Autodesk Inventor part; units mm, degrees
ref_plane "YZ Plane" through (0, 0, 0) normal (1, 0, 0) x (0, 1, 0)
ref_plane "XZ Plane" through (0, 0, 0) normal (0, 1, 0) x (-1, 0, 0)
ref_plane "XY Plane" through (0, 0, 0) normal (0, 0, 1) x (1, 0, 0)
sketch "Sketch1" plane through (0, 0, 0) normal (0, 0, 1) x (1, 0, 0)
  line L0 (0, 0) -> (25, 0)
  line L1 (25, 0) -> (25, 3)
  line L2 (25, 3) -> (0, 3)
  line L3 (0, 3) -> (0, 0)
  dimension "d0" = 25
  dimension "d1" = 3
extrude "Extrusion1" add sketch "Sketch1" along normal blind 450
sketch "Sketch2" plane through (0, 3, 0) normal (0, 1, 0) x (1, 0, 0)
  line L0 (0, 0) -> (0, -450)
  line L1 (0, 0) -> (250, 0)
  line L2 (250, 0) -> (250, -25)
  line L3 (250, -25) -> (0, -25)
  line L4 (0, -25) -> (0, 0)
  dimension "d4" = 250
  dimension "d5" = 25
extrude "Extrusion2" add sketch "Sketch2" along normal blind 3
sketch "Sketch3" plane through (0, 3, 450) normal (0, 1, 0) x (1, 0, 0)
  line L0 (0, 450) -> (0, 0)
  line L1 (0, 0) -> (250, 0)
  line L2 (250, 0) -> (250, 25)
  line L3 (250, 25) -> (0, 25)
  line L4 (0, 25) -> (0, 0)
  dimension "d8" = 250
  dimension "d9" = 25
extrude "Extrusion3" add sketch "Sketch3" along normal blind 3
sketch "Sketch4" plane through (0, 3, 0) normal (0, -1, 0) x (1, 0, 0)
  line L0 (250, 0) -> (0, 0)
  line L1 (250, 0) -> (225, 0)
  line L2 (225, 0) -> (225, 450)
  line L3 (225, 450) -> (250, 450)
  line L4 (250, 450) -> (250, 0)
  dimension "d12" = 25
  dimension "d13" = 450
extrude "Extrusion4" add sketch "Sketch4" along normal blind 3
sketch "Sketch5" plane through (0, 3, 25) normal (0, 1, 0) x (1, 0, 0)
  line L0 (0, 25) -> (0, -175)
  line L1 (0, 0) -> (0, -400)
  line L2 (0, -175) -> (250, -175)
  line L3 (250, -175) -> (250, -225)
  line L4 (250, -225) -> (0, -225)
  line L5 (0, -225) -> (0, -175)
  dimension "d16" = 200
  dimension "d17" = 250
  dimension "d18" = 50
extrude "Extrusion5" add sketch "Sketch5" along normal blind 3
sketch "Sketch6" plane through (0, 6, 0) normal (0, 1, 0) x (1, 0, 0)
  line L0 (25, -25) -> (0, -25)
  line L1 (0, 0) -> (0, -25)
  line L2 (25, -25) -> (0, -25)
  line L3 (0, -25) -> (0, 0)
  line L4 (0, 0) -> (25, 0)
  line L5 (25, 0) -> (25, -25)
  line L6 (25, -25) -> (0, 0)
  line L7 (225, 0) -> (25, 0)
  line L8 (25, 0) -> (0, -25)
  circle A0 centre (12.5, -12.5) radius 2.5
  line L9 (0, -450) -> (250, -450)
  line L10 (250, -425) -> (0, -425)
  line L11 (0, -450) -> (25, -450)
  line L12 (25, -450) -> (25, -425)
  line L13 (25, -425) -> (0, -425)
  line L14 (0, -425) -> (0, -450)
  line L15 (250, -450) -> (225, -450)
  line L16 (225, -450) -> (225, -425)
  line L17 (225, -425) -> (250, -425)
  line L18 (250, -425) -> (250, -450)
  line L19 (0, -450) -> (25, -425)
  line L20 (25, -450) -> (0, -425)
  line L21 (250, -450) -> (225, -425)
  line L22 (225, -425) -> (225, -250)
  line L23 (225, -450) -> (250, -425)
  circle A1 centre (237.5, -437.5) radius 2.5
  circle A2 centre (12.5, -437.5) radius 2.5
  line L24 (250, -25) -> (250, 0)
  line L25 (225, -25) -> (250, -25)
  line L26 (250, 0) -> (225, 0)
  line L27 (225, 0) -> (225, -25)
  line L28 (225, -25) -> (250, -25)
  line L29 (250, -25) -> (250, 0)
  line L30 (250, -25) -> (225, 0)
  line L31 (225, 0) -> (225, -25)
  line L32 (225, 0) -> (225, -25)
  line L33 (225, -25) -> (250, 0)
  circle A3 centre (237.5, -12.5) radius 2.5
  dimension "d21" = 5
  dimension "d22" = 5
  dimension "d23" = 5
  dimension "d24" = 5
extrude "Extrusion6" cut sketch "Sketch6" against normal blind 100 contours A0 L8 L6 | L6 L8 A0 | A0 L6 L8 | L8 L6 A0 | A3 L33 L30 | L30 L33 A3 | A3 L30 L33 | L33 L30 A3 | A2 L20 L19 | L19 L20 A2 | L20 L19 A2 | A2 L19 L20 | A1 L21 L23 | L23 L21 A1 | L21 L23 A1 | A1 L23 L21
sketch "Sketch7" plane through (0, 6, 25) normal (0, 1, 0) x (1, 0, 0)
  circle A0 centre (12.5, -200) radius 2.5
  line L0 (0, -175) -> (0, -225)
  line L1 (0, -225) -> (250, -225)
  circle A1 centre (237.5, -200) radius 2.5
  line L2 (250, -225) -> (250, -175)
  line L3 (250, -175) -> (0, -175)
  point P0 (0, 25)
  dimension "d27" = 5
  dimension "d28" = 12.5
  dimension "d29" = 25
  dimension "d30" = 5
  dimension "d31" = 12.5
  dimension "d32" = 25
extrude "Extrusion7" cut sketch "Sketch7" against normal blind 100 contours A0 | A1
thread "Thread1"
thread "Thread2"
thread "Thread3"
thread "Thread4"
thread "Thread5"
thread "Thread6"
sketch "Sketch8" plane through (0, 6, 25) normal (0, 1, 0) x (1, 0, 0)
  circle A0 centre (12.5, -200) radius 2.5
  circle A1 centre (237.5, -200) radius 2.5
  circle A2 centre (125, -200) radius 6.35
  line L0 (250, -225) -> (250, -175)
  point P0 (0, 25)
  dimension "d47" = 12.7
  dimension "d48" = 125
extrude "Extrusion8" cut sketch "Sketch8" against normal blind 10 contours A2
sketch "Sketch9" plane through (0, 6, 450) normal (0, 1, 0) x (1, 0, 0)
  circle A0 centre (125, 11.2801) radius 6.35
  line L0 (250, 0) -> (250, 25)
  point P0 (0, 450)
  dimension "d51" = 12.7
  dimension "d52" = 125
extrude "Extrusion9" cut sketch "Sketch9" against normal through all
thread "Thread7"
sketch "Sketch10" plane through (0, 3, 425) normal (0, 1, 0) x (1, 0, 0)
  line L0 (25, 425) -> (25, -25)
  line L1 (0, 425) -> (0, -25)
  line L2 (25, 0.3749) -> (0, 0.3749)
  line L3 (0, 0.3749) -> (0, 100.3749)
  line L4 (0, 100.3749) -> (25, 100.3749)
  line L5 (25, 100.3749) -> (25, 0.3749)
  circle A0 centre (12.5, 20.3749) radius 2.5
  circle A1 centre (12.5, 80.3749) radius 2.5
  point P0 (12.5, 0.3749)
  point P1 (12.5, 100.3749)
  dimension "d57" = 100
  dimension "d58" = 5
  dimension "d59" = 5
  dimension "d60" = 20
  dimension "d61" = 20
  dimension "d62" = 12.5
  dimension "d63" = 12.5
extrude "Extrusion10" cut sketch "Sketch10" against normal blind 10 contours A0 | A1
thread "Thread8"
thread "Thread9"
properties part number "Base Platform"
Here's how the part is built. I have some questions about the finished solid (model axes, mm). A direction names the side the tool comes from. Round coordinates to 2 decimals unless told otherwise and drop trailing zeros. Loops run counter-clockwise (first coordinate to the right, second up) from the corner with the lowest first, then second, coordinate; pieces in that order, holes last.
1. If we section it at B-B on z = 34.5: Write out the boundary of the cut face in (x, y).
Answer list:
outline: (0, 0) - (25, 0) - (25, 3) - (0, 3) - close; (225, 0) - (250, 0) - (250, 3) - (225, 3) - close
2. If we section it at D-D on y = 0.9: Count the separate pieces of the cut face and the enclosed holes in it, plus the area to 3 significant figures.
Answer list:
separate pieces: 2
enclosed holes: 8
area: 22,300 mm2
3. If we section it at A-A on x = 125: Write out the boundary of the cut face in (y, z).
Answer list:
outline: (3, 0) - (6, 0) - (6, 25) - (3, 25) - close; (3, 200) - (6, 200) - (6, 218.65) - (3, 218.65) - close; (3, 231.35) - (6, 231.35) - (6, 250) - (3, 250) - close; (3, 425) - (6, 425) - (6, 432.37) - (3, 432.37) - close; (3, 445.07) - (6, 445.07) - (6, 450) - (3, 450) - close
4. We'd pull the mould along Z, two halves only. Please class faces 1 (the face through (237, 3, 114)), 2 (the face through (123, 6, 236)), 3 (the face through (13, 3, 111)): +Z half, -Z half, draft (parallel to the pull), parting line (faces both ways), or undercut.
Answer list:
face 1: undercut
face 2: draft
face 3: undercut
5. Which directions (+Z, -Z, +X, -X, +Y, -Y) give clear straight access to the entire face, cutting with the end or side of a thin tool? Please do faces 4 (the face through (123, 6, 432)), 5 (the face through (124, 3, 12)), 6 (the face through (13, 3, 336)).
Answer list:
face 4: +Z, -Z, +X, -X, +Y
face 5: +Z, -Z, -Y
face 6: +X, -X, +Y
6. If I drill on line 1 along X through (y, z) = (3.25, 12.5); line 2 along Z through (x, y) = (210, 4.1); line 3 along Z through (x, y) = (125, 5.4), over which ranges is the centre line in solid material (lowest first)?
Answer list:
line 1: x = 0 to 10, 15 to 235, 240 to 250
line 2: z = 0 to 25, 200 to 250, 425 to 450
line 3: z = 0 to 25, 200 to 218.65, 231.35 to 250, 425 to 432.37, 445.07 to 450
7. If we section it at C-C on x = 159: Write out the boundary of the cut face in (y, z), plus the area to 3 significant figures.
Answer list:
outline: (3, 0) - (6, 0) - (6, 25) - (3, 25) - close; (3, 200) - (6, 200) - (6, 250) - (3, 250) - close; (3, 425) - (6, 425) - (6, 450) - (3, 450) - close
area: 300 mm2
8. For P1, Ø12.5, axis at x = 108.5, z = 17, coming from the -Y side; P2, Ø1.5, axis at x = 161.5, y = 5, coming from the -Z side, each with a flat end and sliding along its axis, tell me the tip position at first contact or that it passes through.
Answer list:
P1: stops at y = 3
P2: stops at z = 0
